```python
from build123d import *

# Parameters (mm, degrees)
F2_T = -2.5


with BuildPart() as f1:
    # F0 (on Top) → F1 (revolve)
    with BuildSketch(Plane.XY):
        Polygon((29.168965295, 20.9186449647), (0, 20.9186449647), (0, -55.4267726839), (19.8249841153, -55.4267726839), (25.6272411018, 0), (29.168965295, 1.331854861), align=None)
    revolve(axis=Axis((0, 0.3053806722, 0), (0, -1, 0)))

    # F2
    f2_openings = [f1.faces().sort_by_distance(p)[0] for p in [
        (0, 20.918645, 0),
    ]]
    offset(amount=F2_T, openings=f2_openings, kind=Kind.INTERSECTION)


solid = f1.part
```
The listing builds one solid part. Answer for the finished solid, in the listing's coordinates (mm). Round coordinates to 2 decimals unless told otherwise and drop trailing zeros. Write each loop counter-clockwise with the first axis right and the second up, starting at its lowest first coordinate (ties: lowest second). Pieces come first, ordered by that corner, then holes. Notation, with made-up numbers: (15.5, 49) -> (63.5, 49) arc R28 cw to (63.5, 88) -> close; hole circle Ø10 at (4, 47.25). An arc over 180 degrees is marked (long way). Answer as a JSON object with one key per item and string values. Group by question number.
Q1. Determine the mould class of faces 1 (the face through (0, -52.927, 0)), 2 (the face through (-5.781, 12.116, -26.035)), 3 (the face through (-6.323, 11.262, -28.475)), 4 (the face through (0, -55.427, 0)) for opening direction Z: pulls with the +Z half, pulls with the -Z half, needs draft (parallel to the pull), parting line crosses it, or undercut.
Q2. Section B-B (x = 0) is taken. Write down the section's boundary in (y, z), plus the area to 3 significant figures.
Q3. Section C-C (y = 12) is taken. Write down the section's boundary in (x, z), plus the area to 3 significant figures.
Q4. Section D-D (y = -18) is taken. Write down the section's boundary in (x, z).
Q5. Section A-A (z = 0) is taken. Write down the section's boundary in (x, y), plus the area to 3 significant figures.
Q6. Each of these flat-tipped pins is pushed along its axis until it touches: pin 1 Ø5 at (x, y) = (18.5, 10) entering from +Z; pin 2 Ø10.5 at (x, z) = (1, -1) entering from +Y; pin 3 Ø12 at (y, z) = (-7.5, 9) entering from +X. Where does it stop, or does it pass through?
Q7. Straight lines are drawn through the part: line 1 along Z through (x, y) = (0, 7); line 2 along Y through (x, z) = (-7, 3); line 3 along Z through (x, y) = (-12, 14). For each, find the intervals that lie inside material, in ascending order.
Check values:
{
 "1": {"face 1": "undercut", "face 2": "undercut", "face 3": "parting line crosses it", "face 4": "needs draft"},
 "2": {"outline": "(-55.43, -19.82) -> (0, -25.63) -> (1.33, -29.17) -> (20.92, -29.17) -> (20.92, -26.67) -> (3.06, -26.67) -> (1.8, -23.3) -> (-52.93, -17.57) -> (-52.93, 17.57) -> (1.8, 23.3) -> (3.06, 26.67) -> (20.92, 26.67) -> (20.92, 29.17) -> (1.33, 29.17) -> (0, 25.63) -> (-55.43, 19.82) -> close", "area": "482 mm^2"},
 "3": {"outline": "circle Ø58.34 at (0, 0); hole circle Ø53.34 at (0, 0)", "area": "439 mm^2"},
 "4": {"outline": "circle Ø47.49 at (0, 0); hole circle Ø42.46 at (0, 0)"},
 "5": {"outline": "(-29.17, 1.33) -> (-25.63, 0) -> (-19.82, -55.43) -> (19.82, -55.43) -> (25.63, 0) -> (29.17, 1.33) -> (29.17, 20.92) -> (26.67, 20.92) -> (26.67, 3.06) -> (23.3, 1.8) -> (17.57, -52.93) -> (-17.57, -52.93) -> (-23.3, 1.8) -> (-26.67, 3.06) -> (-26.67, 20.92) -> (-29.17, 20.92) -> close", "area": "482 mm^2"},
 "6": {"pin 1": "z = 24.39", "pin 2": "y = -52.93", "pin 3": "x = 24.87"},
 "7": {"line 1": "-29.17 to -26.67, 26.67 to 29.17", "line 2": "-55.43 to -52.93", "line 3": "-26.59 to -23.82, 23.82 to 26.59"}
}
